from build123d import *

# Parameters (mm, degrees)
F0_W      = 92
F0_H      = 92
F1_DEPTH  = 5.25
F1_FACE_W = 92
F1_FACE_H = 92
F5_R      = 10.75
F6_W      = 66.25
F6_H      = 66.25
F7_DEPTH  = 13
F8_R      = 1


with BuildPart() as f1:
    # F0 (on Top) → F1 (new body)
    with BuildSketch(Plane.XY):
        Rectangle(F0_W, F0_H)
    extrude(amount=F1_DEPTH)

    # F1_face (on face) → F4 section 0
    with BuildSketch(Plane.XY.offset(5.25), mode=Mode.PRIVATE) as f4_s0:
        Rectangle(F1_FACE_W, F1_FACE_H)
    loft([f4_s0.sketch, Vertex(0, 0, 15.5)])

    # F5
    f5_edges = [f1.edges().sort_by_distance(p)[0] for p in [
        (-46, -46, 2.625),
        (46, -46, 2.625),
        (46, 46, 2.625),
        (-46, 46, 2.625),
    ]]
    fillet(f5_edges, radius=F5_R)

    # F6 (on face) → F7 (join)
    with BuildSketch(Plane(origin=(0, 0, 0), x_dir=(1, 0, 0), z_dir=(0, 0, -1))):
        Rectangle(F6_W, F6_H)
    extrude(amount=F7_DEPTH)

    # F8
    f8_edges = [f1.edges().sort_by_distance(p)[0] for p in [
        (33.125, 33.125, -6.5),
        (-33.125, 33.125, -6.5),
        (-33.125, -33.125, -6.5),
        (33.125, -33.125, -6.5),
    ]]
    fillet(f8_edges, radius=F8_R)


solid = f1.part
For this review, take the finished solid that the model builds, in its own axes (mm). A direction names the side the tool comes from. Round coordinates to 2 decimals unless told otherwise and drop trailing zeros. Loops run counter-clockwise (first coordinate to the right, second up) from the corner with the lowest first, then second, coordinate; pieces in that order, holes last. Notation, with made-up numbers: (-1.5, 64.5) - (5.5, 64.5) arc R15 cw to (5.5, 76.5) - close; hole circle Ø4 at (3.5, -19). An arc over 180 degrees is marked (long way). One line per question, with ' | ' between items.
Q1. Take a section at C-C (z = -8). Give the boundary of the cut face in (x, y) (3 decimals), and give its area (3 significant figures).
Taken from the geometry:
outline: (-33.125, -32.125) arc R1 ccw to (-32.125, -33.125) - (32.125, -33.125) arc R1 ccw to (33.125, -32.125) - (33.125, 32.125) arc R1 ccw to (32.125, 33.125) - (-32.125, 33.125) arc R1 ccw to (-33.125, 32.125) - close | area: 4,390 mm²
Q2. For pin 1 (4 mm diameter, centred on x = -8.5, z = -7, fed in from -Y) (3 decimals); pin 2 (6.5 mm diameter, centred on x = 14.5, z = -9.5, fed in from +Y) (3 decimals); pin 3 (6.5 mm diameter, centred on y = -14, z = -3.5, fed in from +X) (3 decimals), all flat-tipped, find the tip position at first contact; note any pin that passes through.
Taken from the geometry:
pin 1: stops at y = -33.125 | pin 2: stops at y = 33.125 | pin 3: stops at x = 33.125
Q3. Tool access review of faces 1 (the flat face through (33.125, 0, -6)), 2 (the flat face through (0, 33.125, -6)), 3 (the flat face through (0, -33.125, -6)): name each direction out of +Z, -Z, +X, -X, +Y, -Y from which nothing blocks a thin tool from reaching the whole face with its end or side.
Taken from the geometry:
face 1: -Z, +X, +Y, -Y | face 2: -Z, +X, -X, +Y | face 3: -Z, +X, -X, -Y
Q4. For line 1 along Y through (x, z) = (-19.5, -2.5) (3 decimals); line 2 along Z through (x, y) = (-41.5, -35), list the stretches that pass through material, from the lowest coordinate up. Write a range as [from, to].
Taken from the geometry:
line 1: y = [-33.125, 33.125] | line 2: z = [0, 6.25]
Q5. Take a section at A-A (y = 14). Give the boundary of the cut face in (x, z) (3 decimals).
Taken from the geometry:
outline: (-46, 0) - (-33.125, 0) - (-33.125, -13) - (33.125, -13) - (33.125, 0) - (46, 0) - (46, 5.25) - (14, 12.38) - (-14, 12.38) - (-46, 5.25) - close
Q6. Take a section at D-D (x = -37). Give the boundary of the cut face in (y, z), and give its area (3 significant figures).
Taken from the geometry:
outline: (-45.86, 0) - (45.86, 0) - (45.86, 5.28) - (37, 7.26) - (-37, 7.26) - (-45.86, 5.28) - close | area: 648 mm²
Q7. Take a section at B-B (x = 9). Give the boundary of the cut face in (y, z) (3 decimals), and give its area (3 significant figures).
Taken from the geometry:
outline: (-46, 0) - (-33.125, 0) - (-33.125, -13) - (33.125, -13) - (33.125, 0) - (46, 0) - (46, 5.25) - (9, 13.495) - (-9, 13.495) - (-46, 5.25) - close | area: 1,800 mm²
